from build123d import *

# Parameters (mm, degrees)
SKETCH2_R               = 21.082
SKETCH2_R_2             = 17.526
BOSS_EXTRUDE1_DEPTH     = 587.375
F_1_4_CLEARANCE_HOLE1_D = 7.14248


with BuildPart() as part:
    # Sketch2 → Boss-Extrude1 (new, symmetric)
    with BuildSketch(Plane(origin=(0, 0, 0), x_dir=(1, 0, 0), z_dir=(0, 1, 0))):
        with Locations(Location((0, 0, 0), (0, 0, 270))):
            Circle(SKETCH2_R)
        with Locations(Location((0, 0, 0), (0, 0, 270))):
            Circle(SKETCH2_R_2, mode=Mode.SUBTRACT)
    extrude(amount=BOSS_EXTRUDE1_DEPTH, both=True)

    # 1/4 Clearance Hole1 (through all)
    with Locations(Plane(origin=(21.082, 544.83, 0), x_dir=(0, 0, 1), z_dir=(1, 0, 0))):
        with Locations((0, 0), (0, 1089.66)):
            Hole(F_1_4_CLEARANCE_HOLE1_D / 2)


solid = part.part
Design review of the part built by this model. Coordinates are the model's own, in mm. Give positions to 0.01 mm unless a question says otherwise; leave off trailing zeros. Loops run counter-clockwise (first coordinate to the right, second up) from the corner with the lowest first, then second, coordinate; pieces in that order, holes last. Notation, with made-up numbers: M 27.5,-9.75 L 34.5,-9.75 A17 cw 34.5,-5.75 Z; hole C 55,51 d10. An arc over 180 degrees is marked long. Write item = value, one per line.
Q1. Draft analysis for pull direction Z (two halves, no side actions). For faces 1 (the cylindrical face through (-10.66, -8.22, -13.91)), 2 (the flat face through (16, 587.375, -8)), 3 (the cylindrical face through (-8.075, 8.223, 19.474)), state which applies: +Z half, -Z half, draft (parallel to the pull), parting line (faces both ways), or undercut.
Output values:
face_1 = undercut
face_2 = draft
face_3 = parting line
Q2. To check wall thickness, follow line 1 (Y direction, x = 19.55, z = 0) (3 decimals); line 2 (Y direction, x = 18.5, z = -1) (3 decimals); line 3 (X direction, y = -454, z = 0). State the ranges of each line that lie inside material, in increasing order. Write a range as [from, to].
Output values:
line_1 = [-587.375, -548.401], [-541.259, 541.259], [548.401, 587.375]
line_2 = [-587.375, -548.258], [-541.402, 541.402], [548.258, 587.375]
line_3 = [-21.08, -17.53], [17.53, 21.08]
Q3. We need section A-A (x = 0). Give the boundary of the cut face in (y, z) (3 decimals).
Output values:
outline = M -587.375,-21.082 L 587.375,-21.082 L 587.375,-17.526 L -587.375,-17.526 Z; M -587.375,17.526 L 587.375,17.526 L 587.375,21.082 L -587.375,21.082 Z
Q4. We need section B-B (y = -425.5). Give the boundary of the cut face in (x, z).
Output values:
outline = C 0,0 d42.16; hole C 0,0 d35.05
Q5. Insertion check: pin 1 (10 mm diameter, centred on x = -11.5, y = 385.5, fed in from +Z); pin 2 (1.5 mm diameter, centred on y = 423, z = 13.5, fed in from +X); pin 3 (3 mm diameter, centred on x = -6.5, y = 262.5, fed in from +Z). Each pin has a flat end and moves straight along its axis. Give the tip position at first contact, or say it passes through.
Output values:
pin_1 = 20.05
pin_2 = 16.79
pin_3 = 20.48
